Could you check a few things on this model? Use its own coordinates, in mm. A direction names the side the tool comes from. Coordinates: 2 decimals unless noted, no trailing zeros. Write each loop counter-clockwise with the first axis right and the second up, starting at its lowest first coordinate (ties: lowest second). Pieces come first, ordered by that corner, then holes.
Item 1: I want a section at C-C on x = 0.3. Please give me the cut outline in (y, z).
Item 2: For P1, Ø0.5, axis at x = -1, z = 4.5, coming from the -Y side; P2, Ø0.6, axis at y = 13, z = 5.5, coming from the +X side, each with a flat end and sliding along its axis, tell me the tip position at first contact or that it passes through.
Item 3: Thinking about a two-plate mould opening in X: for faces 1 (the flat face through (-2, 3, 3.5)), 2 (the flat face through (2, 3, 3.5)), 3 (the flat face through (-0.75, 7.6, 3.5)), which applies, +X half, -X half, draft (parallel to the pull), parting line (faces both ways), or undercut?
Item 4: If I drill on probe 1 along Y at (x, z) = (-1.35, 2.5); probe 2 along X at (y, z) = (10.25, 0.75); probe 3 along X at (y, z) = (3.25, 3.5), over which ranges is the centre line in solid material (lowest first)?
Item 5: Which directions (+Z, -Z, +X, -X, +Y, -Y) give clear straight access to the entire face, cutting with the end or side of a thin tool? Please do faces 4 (the cylindrical face through (0.014, 11.285, 5.699)), 5 (the flat face through (-0.75, 5.6, 3.5)), 6 (the flat face through (1.4, 7, 3)).
Item 6: I want a section at A-A on y = 4.25. Please give me the cut outline in (x, z), then the cut area to 3 significant figures.
Item 7: I want a section at B-B on y = 12.25. Please give me the cut outline in (x, z).
from build123d import *

# Parameters (mm, degrees)
BOX013_W     = 1
BOX013_H     = 2
BOX013_DEPTH = 2
BOX012_W     = 1
BOX012_H     = 2
BOX012_DEPTH = 2
CHAMFER_SIZE = 0.5
BOX007_W     = 2
BOX007_H     = 2.5
BOX007_DEPTH = 1
BOX008_W     = 2
BOX008_H     = 2.5
BOX008_DEPTH = 1
BOX_W        = 1.5
BOX_H        = 10
BOX_DEPTH    = 7
BOX001_W     = 2.8
BOX001_H     = 1.2
BOX001_DEPTH = 7
BOX002_W     = 2.8
BOX002_H     = 1.2
BOX002_DEPTH = 7
BOX003_W     = 2.8
BOX003_H     = 1.2
BOX003_DEPTH = 7
BOX004_W     = 2.8
BOX004_H     = 1.2
BOX004_DEPTH = 7
BOX005_W     = 2.8
BOX005_H     = 3
BOX005_DEPTH = 7
BOX006_W     = 5
BOX006_H     = 13.5
BOX006_DEPTH = 7
FILLET_R     = 1
FILLET007_R  = 1
FILLET008_R  = 0.4
FILLET009_R  = 0.2


with BuildPart() as cube013:
    # Box013 → Box013 (new body)
    with BuildSketch(Plane(origin=(-3, 2, 2.5), x_dir=(1, 0, 0), z_dir=(0, 0, 1))):
        with Locations((0.5, 1)):
            Rectangle(BOX013_W, BOX013_H)
    extrude(amount=BOX013_DEPTH)


with BuildPart() as chamfer_body:
    # Box012 → Box012 (new body)
    with BuildSketch(Plane(origin=(2, 2, 2.5), x_dir=(1, 0, 0), z_dir=(0, 0, 1))):
        with Locations((0.5, 1)):
            Rectangle(BOX012_W, BOX012_H)
    extrude(amount=BOX012_DEPTH)

    # Fusion005: union Cube013
    add(cube013.part)

    # Chamfer
    chamfer_edges = [chamfer_body.edges().sort_by_distance(p)[0] for p in [
        (2, 2, 3.5),
        (2, 3, 4.5),
        (2, 4, 3.5),
        (2, 3, 2.5),
        (-2, 2, 3.5),
        (-2, 3, 4.5),
        (-2, 4, 3.5),
        (-2, 3, 2.5),
    ]]
    chamfer(chamfer_edges, length=CHAMFER_SIZE)


with BuildPart() as cube007:
    # Box007 → Box007 (new body)
    with BuildSketch(Plane(origin=(-1, 11, 0), x_dir=(1, 0, 0), z_dir=(0, 0, 1))):
        with Locations((1, 1.25)):
            Rectangle(BOX007_W, BOX007_H)
    extrude(amount=BOX007_DEPTH)


with BuildPart() as fusion001:
    # Box008 → Box008 (new body)
    with BuildSketch(Plane(origin=(-1, 11, 6), x_dir=(1, 0, 0), z_dir=(0, 0, 1))):
        with Locations((1, 1.25)):
            Rectangle(BOX008_W, BOX008_H)
    extrude(amount=BOX008_DEPTH)

    # Fusion001: union Cube007
    add(cube007.part)


with BuildPart() as cube:
    # Box → Box (new body)
    with BuildSketch(Plane(origin=(-0.75, 0, 0), x_dir=(1, 0, 0), z_dir=(0, 0, 1))):
        with Locations((0.75, 5)):
            Rectangle(BOX_W, BOX_H)
    extrude(amount=BOX_DEPTH)


with BuildPart() as cube001:
    # Box001 → Box001 (new body)
    with BuildSketch(Plane(origin=(-1.4, 0, 0), x_dir=(1, 0, 0), z_dir=(0, 0, 1))):
        with Locations((1.4, 0.6)):
            Rectangle(BOX001_W, BOX001_H)
    extrude(amount=BOX001_DEPTH)


with BuildPart() as cube002:
    # Box002 → Box002 (new body)
    with BuildSketch(Plane(origin=(-1.4, 2, 0), x_dir=(1, 0, 0), z_dir=(0, 0, 1))):
        with Locations((1.4, 0.6)):
            Rectangle(BOX002_W, BOX002_H)
    extrude(amount=BOX002_DEPTH)


with BuildPart() as cube003:
    # Box003 → Box003 (new body)
    with BuildSketch(Plane(origin=(-1.4, 4, 0), x_dir=(1, 0, 0), z_dir=(0, 0, 1))):
        with Locations((1.4, 0.6)):
            Rectangle(BOX003_W, BOX003_H)
    extrude(amount=BOX003_DEPTH)


with BuildPart() as cube004:
    # Box004 → Box004 (new body)
    with BuildSketch(Plane(origin=(-1.4, 6, 0), x_dir=(1, 0, 0), z_dir=(0, 0, 1))):
        with Locations((1.4, 0.6)):
            Rectangle(BOX004_W, BOX004_H)
    extrude(amount=BOX004_DEPTH)


with BuildPart() as fusion:
    # Box005 → Box005 (new body)
    with BuildSketch(Plane(origin=(-1.4, 8, 0), x_dir=(1, 0, 0), z_dir=(0, 0, 1))):
        with Locations((1.4, 1.5)):
            Rectangle(BOX005_W, BOX005_H)
    extrude(amount=BOX005_DEPTH)

    # Fusion: union Cube, Cube001, Cube002, Cube003, Cube004
    add(cube.part)
    add(cube001.part)
    add(cube002.part)
    add(cube003.part)
    add(cube004.part)


with BuildPart() as fillet009:
    # Box006 → Box006 (new body)
    with BuildSketch(Plane(origin=(-2.5, 0, 0), x_dir=(1, 0, 0), z_dir=(0, 0, 1))):
        with Locations((2.5, 6.75)):
            Rectangle(BOX006_W, BOX006_H)
    extrude(amount=BOX006_DEPTH)

    # Cut: cut Fusion
    add(fusion.part, mode=Mode.SUBTRACT)

    # Cut004: cut Fusion001
    add(fusion001.part, mode=Mode.SUBTRACT)

    # Cut005: cut Chamfer body
    add(chamfer_body.part, mode=Mode.SUBTRACT)

    # Fillet
    fillet_edges = [fillet009.edges().sort_by_distance(p)[0] for p in [
        (0, 13.5, 1),
        (0, 13.5, 6),
        (0, 11, 1),
        (0, 11, 6),
    ]]
    fillet(fillet_edges, radius=FILLET_R)

    # Fillet007
    fillet007_edges = [fillet009.edges().sort_by_distance(p)[0] for p in [
        (-2.5, 13.5, 3.5),
        (2.5, 13.5, 3.5),
    ]]
    fillet(fillet007_edges, radius=FILLET007_R)

    # Fillet008
    fillet008_edges = [fillet009.edges().sort_by_distance(p)[0] for p in [
        (-1.4, 0, 3.5),
        (1.4, 0, 3.5),
    ]]
    fillet(fillet008_edges, radius=FILLET008_R)

    # Fillet009
    fillet009_edges = [fillet009.edges().sort_by_distance(p)[0] for p in [
        (-2.5, 0, 3.5),
        (2.5, 0, 3.5),
    ]]
    fillet(fillet009_edges, radius=FILLET009_R)


solid = fillet009.part
Response values:
1. outline: (11, 2) arc R1 ccw to (12, 1) - (12.5, 1) arc R1 ccw to (13.5, 2) - (13.5, 5) arc R1 ccw to (12.5, 6) - (12, 6) arc R1 ccw to (11, 5) - close
2. P1: stops at y = 1.2
2. P2: stops at x = 2.48
3. face 1: -X half
3. face 2: +X half
3. face 3: undercut
4. probe 1: y = 1.2 to 2, 3.2 to 4, 5.2 to 6, 7.2 to 8, 11 to 13.5
4. probe 2: x = -2.5 to -1.4, 1.4 to 2.5
4. probe 3: x = -2 to -0.75, 0.75 to 2
5. face 4: +Z
5. face 5: +Z, -Z, -Y
5. face 6: +Z, -Z
6. outline: (-2.5, 0) - (-1.4, 0) - (-1.4, 7) - (-2.5, 7) - close; (1.4, 0) - (2.5, 0) - (2.5, 7) - (1.4, 7) - close
6. area: 15.4 mm2
7. outline: (-2.5, 0) - (-1, 0) - (-1, 1) - (1, 1) - (1, 0) - (2.5, 0) - (2.5, 7) - (1, 7) - (1, 6) - (-1, 6) - (-1, 7) - (-2.5, 7) - close
